from build123d import *

# Parameters (mm, degrees)
SKETCH037_W       = 7.5
SKETCH037_H       = 7.5
EXTRUDE045_DEPTH  = 10
SKETCH036_W       = 10
SKETCH036_H       = 9
EXTRUDE044_DEPTH  = 10
CYLINDER001_R     = 2
CYLINDER001_DEPTH = 10
SKETCH032_R       = 2.6
EXTRUDE043_DEPTH  = 0.8
EXTRUDE055_DEPTH  = 3
EXTRUDE056_DEPTH  = 0.8
EXTRUDE038_DEPTH  = 2


with BuildPart() as extrude045:
    # Sketch037 → Extrude045 (new body)
    with BuildSketch(Plane.YZ.offset(35)):
        with Locations((0, 8)):
            Rectangle(SKETCH037_W, SKETCH037_H)
    extrude(amount=EXTRUDE045_DEPTH)


with BuildPart() as extrude045_1:
    # Extrude045 placement: moved
    add(extrude045.part.moved(Location((-9.5, 0, 0))))


with BuildPart() as extrude044:
    # Sketch036 → Extrude044 (new body)
    with BuildSketch(Plane.XY.offset(40)):
        Rectangle(SKETCH036_W, SKETCH036_H)
    extrude(amount=EXTRUDE044_DEPTH)


with BuildPart() as extrude044_1:
    # Extrude044 placement: moved
    add(extrude044.part.moved(Location((0, 0, -15.5))))


with BuildPart() as common_sub:
    # Cylinder001 → Cylinder001 (new body)
    with BuildSketch(Plane(origin=(-92.5, 0, 12), x_dir=(0, 0, 1), z_dir=(-1, 0, 0))):
        Circle(CYLINDER001_R)
    extrude(amount=CYLINDER001_DEPTH)

    # Fusion033: union Extrude045, Extrude044
    add(extrude045_1.part)
    add(extrude044_1.part)


with BuildPart() as sweep_body:
    # Sweep: sweep along a path in Sketch034
    with BuildLine(Plane.XZ.offset(10)) as sweep_path:
        Line((32, 11.999174), (32, 26.4))
        ThreePointArc((32, 26.4), (30.652691, 29.652691), (27.4, 31))
        Line((27.4, 31), (-60.9, 31))
    # Sketch033 → Sweep (sweep)
    with BuildSketch(Plane.YZ):
        Polygon((-5.3, 29.4), (-3.7, 31), (-3.7, 32), (-6, 32), (-6, 29.4), align=None)
    sweep(path=sweep_path.line)


with BuildPart() as fusion:
    # Sketch032 → Extrude043 (new body)
    with BuildSketch(Plane.XZ.offset(10)):
        with Locations((27.4, 26.4)):
            Circle(SKETCH032_R)
    extrude(amount=EXTRUDE043_DEPTH)


with BuildPart() as fusion_1:
    # Extrude043 placement: moved
    add(fusion.part.moved(Location((0, 5.5, 0))))

    # Fusion: union Sweep body
    add(sweep_body.part)


with BuildPart() as screw_hole_bottom002:
    # Sketch003 → Revolve (revolve)
    with BuildSketch(Plane.XY):
        Polygon((1.6, 3), (1.6, 2), (0, 2), (0, 1.8), (2.6, 1.8), (2.6, 0), (4.6, 0), (4.6, 3), align=None)
    revolve(axis=Axis((0, 0, 0), (0, 1, 0)))


with BuildPart() as screw_hole_bottom002_1:
    # Body003 placement: moved
    add(screw_hole_bottom002.part.moved(Location((27.4, -4.5, 26.4))))


with BuildPart() as bottom010:
    # Sketch053 → Extrude055 (new body)
    with BuildSketch(Plane.XZ.offset(10)):
        with BuildLine():
            ThreePointArc((32, 26.4), (30.652691, 29.652691), (27.4, 31))
            Line((27.4, 31), (-20.9, 31))
            Line((-20.9, 31), (-20.9, 29))
            Line((-20.9, 29), (27.4, 29))
            ThreePointArc((30, 26.4), (29.238478, 28.238478), (27.4, 29))
            Line((30, 12), (30, 26.4))
            Line((32, 12), (30, 12))
            Line((32, 26.4), (32, 12))
        make_face()
    extrude(amount=EXTRUDE055_DEPTH)


with BuildPart() as bottom010_1:
    # Extrude055 placement: moved
    add(bottom010.part.moved(Location((0, 8.5, 0))))


with BuildPart() as bottom011:
    # Sketch052 → Extrude056 (new body)
    with BuildSketch(Plane.XZ.offset(10)):
        with BuildLine():
            ThreePointArc((32, 26.399909), (30.652691, 29.6526), (27.4, 30.999909))
            Line((27.4, 30.999909), (-20.9, 30.999909))
            Line((-20.9, 30.999909), (-20.9, 11.999909))
            Line((-20.9, 11.999909), (32, 11.999909))
            Line((32, 26.399909), (32, 11.999909))
        make_face()
    extrude(amount=EXTRUDE056_DEPTH)


with BuildPart() as bottom011_1:
    # Extrude056 placement: moved
    add(bottom011.part.moved(Location((0, 5.5, 0))))


with BuildPart() as bottom:
    # Sketch030 → Extrude038 (new body)
    with BuildSketch(Plane.XZ.offset(10)):
        with BuildLine():
            ThreePointArc((32, 26.4), (30.652691, 29.652691), (27.4, 31))
            Line((27.4, 31), (-20.9, 31))
            Line((-20.9, 31), (-20.9, 30.1))
            Line((-20.9, 30.1), (27.4, 30.1))
            ThreePointArc((31.1, 26.4), (30.016295, 29.016295), (27.4, 30.1))
            Line((31.1, 12), (31.1, 26.4))
            Line((32, 12), (31.1, 12))
            Line((32, 26.4), (32, 12))
        make_face()
    extrude(amount=EXTRUDE038_DEPTH)


with BuildPart() as bottom_1:
    # Extrude038 placement: moved
    add(bottom.part.moved(Location((0, 10.5, 0))))

    # Fusion029: union screw hole bottom002, bottom010, bottom011
    add(screw_hole_bottom002_1.part)
    add(bottom010_1.part)
    add(bottom011_1.part)

    # Cut: cut Fusion
    add(fusion_1.part, mode=Mode.SUBTRACT)


with BuildPart() as bottom007:
    # Part__Mirroring004: instance of bottom
    add(bottom_1.part.mirror(Plane(origin=(0, 0, 12), x_dir=(0, 1, 0), z_dir=(0, 0, 1))))

    # Fusion031: union bottom
    add(bottom_1.part)

    # Cut026: cut common sub
    add(common_sub.part, mode=Mode.SUBTRACT)


solid = bottom007.part
Check sheet for the modelled part. Datum: model origin and axes. Units: mm. A direction names the side the tool comes from. Coordinates: 2 decimals unless noted, no trailing zeros. Loops run counter-clockwise (first coordinate to the right, second up) from the corner with the lowest first, then second, coordinate; pieces in that order, holes last. Notation, with made-up numbers: (2, 71) -> (15, 71) arc R18 ccw to (15, 84) -> close; hole circle Ø3 at (-39, -22). An arc over 180 degrees is marked (long way). Answer in a Markdown table with one row per item.
1. Go/stop test with flat-tipped pins: pin 1 (3.5 mm diameter, centred on x = 28, z = -2.5, fed in from +Y); pin 2 (1 mm diameter, centred on y = -0.5, z = 0.5, fed in from -X); pin 3 (1 mm diameter, centred on x = 31.5, y = -1.5, fed in from -Z). Record where each tip stops, or that it passes through.
Check values:
| item | result |
|---|---|
| pin 1 | stops at y = -1.5 |
| pin 2 | stops at x = 31.1 |
| pin 3 | stops at z = -5.26 |
2. Sectioned sample at C-C, the plane z = 10. Record the boundary of the cut face in (x, y).
Check values:
| item | result |
|---|---|
| outline | (-20.9, -5.3) -> (30.4, -5.3) -> (31.95, -3.75) -> (30, -3.75) -> (30, -4.5) -> (-20.9, -4.5) -> close |
3. Material ranges on line 1 along Z through (x, y) = (27.4, -3.45); line 2 along Z through (x, y) = (27.4, -4.4); line 3 along Z through (x, y) = (23, -0.15), recorded low to high. Write a range as [from, to].
Check values:
| item | result |
|---|---|
| line 1 | z = [-7, -5], [0.2, 2.2], [21.8, 23.8], [29, 31] |
| line 2 | z = [-6.3, -5], [0.2, 2.2], [21.8, 23.8], [29, 30.3] |
| line 3 | z = [-7, -6.1], [30.1, 31] |
4. Sectioned sample at D-D, the plane x = 11. Record the boundary of the cut face in (y, z).
Check values:
| item | result |
|---|---|
| outline | (-5.3, -5.4) -> (-3.7, -7) -> (0.5, -7) -> (0.5, -6.1) -> (-1.5, -6.1) -> (-1.5, -5) -> (-4.5, -5) -> (-4.5, 29) -> (-1.5, 29) -> (-1.5, 30.1) -> (0.5, 30.1) -> (0.5, 31) -> (-3.7, 31) -> (-5.3, 29.4) -> close |
5. Access from +Z, -Z, +X, -X, +Y, -Y to the whole of each face (thin tool, end or side, straight path). Record for faces 4 (the face through (31, -2, 4.25)), 5 (the face through (29.88, -3.98, 27.18)), 6 (the face through (30.04, -0.49, 28.99)), 7 (the face through (28.926, -2.007, 25.919)).
Check values:
| item | result |
|---|---|
| face 4 | +X, -X, +Y |
| face 5 | -Y |
| face 6 | -X, +Y |
| face 7 | +Y |
6. Sectioned sample at B-B, the plane x = -4. Record the boundary of the cut face in (y, z).
Check values:
| item | result |
|---|---|
| outline | (-5.3, -5.4) -> (-3.7, -7) -> (0.5, -7) -> (0.5, -6.1) -> (-1.5, -6.1) -> (-1.5, -5) -> (-4.5, -5) -> (-4.5, 30.2) -> (-5.3, 29.4) -> close |
7. Sectioned sample at A-A, the plane y = -0.2. Record the boundary of the cut face in (x, z).
Check values:
| item | result |
|---|---|
| outline | (-20.9, -7) -> (27.4, -7) arc R4.6 ccw to (32, -2.4) -> (32, 4.25) -> (31.1, 4.25) -> (31.1, -2.4) arc R3.7 cw to (27.4, -6.1) -> (-20.9, -6.1) -> close; (-20.9, 30.1) -> (-5, 30.1) -> (-5, 31) -> (-20.9, 31) -> close; (5, 30.1) -> (27.4, 30.1) arc R3.7 cw to (31.1, 26.4) -> (31.1, 11.75) -> (32, 11.75) -> (32, 26.4) arc R4.6 ccw to (27.4, 31) -> (5, 31) -> close |
8. Release check for a two-part mould opening along Z. For faces 1 (the face through (32, -2, 1)), 2 (the face through (30, -3, 14)), 3 (the face through (16, -2, 31)) record: released by +Z, released by -Z, zero draft, split by the parting line, or undercut.
Check values:
| item | result |
|---|---|
| face 1 | zero draft |
| face 2 | undercut |
| face 3 | released by +Z |
